Read the model definition and answer for the solid it produces. Units are mm, in the model's axes. A direction names the side the tool comes from. Round coordinates to 2 decimals unless told otherwise and drop trailing zeros. Loops run counter-clockwise (first coordinate to the right, second up) from the corner with the lowest first, then second, coordinate; pieces in that order, holes last. Notation, with made-up numbers: (41.25, -27.5) - (66.25, -27.5) arc R28 ccw to (66.25, 7.5) - close; hole circle Ø11 at (-31.5, 20). An arc over 180 degrees is marked (long way). Use CSV: the item, a comma, the result in double quotes. Start each with the question number.
1. Find section A-A (z = -17). Give the vertices of the cut face in (x, y).
2. Find section B-B (x = 21.5). Give the vertices of the cut face in (y, z).
3. Given pin 1 Ø16.5 at (x, z) = (-16.5, 6.5) entering from -Y, flat-ended and moving along its own axis, determine where the tip first touches the part or whether it passes through.
4. A tool of negligible diameter and unlimited length cuts with its end or side. For faces 1 (the cylindrical face through (7.246, -2.522, -7.744)), 2 (the flat face through (1, 0, -9)), from which of +Z, -Z, +X, -X, +Y, -Y can it reach the whole face along a straight path? Write none if from no direction.
5. Find section D-D (x = -29). Give the vertices of the cut face in (y, z).
6. Find section C-C (z = -34.5). Give the vertices of the cut face in (x, y).
7. Consider line 1 along Z through (x, y) = (8, -1.7); line 2 along X through (y, z) = (-2.4, -21.5); line 3 along Z through (x, y) = (-17.5, -2.7). Determine where each line is inside the solid, lowest interval first.
from build123d import *

# Parameters (mm, degrees)
F0_W     = 76.2
F0_H     = 101.6
F1_DEPTH = 2.54
F2_W     = 33.02
F2_H     = 88.9
F3_DEPTH = 1.27
F4_W     = 17.78
F4_H     = 17.78
F5_DEPTH = 2.54
F6_R     = 2.54
F7_DEPTH = 2.54


with BuildPart() as f1:
    # F0 (on Front) → F1 (new body)
    with BuildSketch(Plane.XZ):
        with Locations((1.335782, -9.618688)):
            Rectangle(F0_W, F0_H)
    extrude(amount=F1_DEPTH)

    # F2 (on face) → F3 (cut)
    with BuildSketch(Plane.XZ.offset(2.54)):
        with Locations((-17.679934, -7.495851)):
            Rectangle(F2_W, F2_H)
        with Locations((20.525211, -7.666058)):
            Rectangle(F2_W, F2_H)
    extrude(amount=-F3_DEPTH, mode=Mode.SUBTRACT)

    # F4 (on face) → F5 (join)
    with BuildSketch(Plane.XZ.offset(1.27)):
        with Locations((-17.624406, 20.281628)):
            Rectangle(F4_W, F4_H)
        with Locations((-17.073924, -4.828554)):
            Rectangle(F4_W, F4_H)
        with Locations((-16.956719, -29.41318)):
            Rectangle(F4_W, F4_H)
        with Locations((20.393534, 20.128676)):
            Rectangle(F4_W, F4_H)
        with Locations((20.905885, -5.264044)):
            Rectangle(F4_W, F4_H)
        with Locations((21.396337, -29.502603)):
            Rectangle(F4_W, F4_H)
    extrude(amount=F5_DEPTH)

    # F6 (on face) → F7 (join)
    with BuildSketch(Plane.XZ.offset(1.27)):
        with Locations((-4.850546, -5.14735)):
            Circle(F6_R)
        with Locations((7.796882, -5.264044)):
            Circle(F6_R)
    extrude(amount=F7_DEPTH)


solid = f1.part
Filled sheet:
1,outline,"(-36.76, -2.54) - (-34.19, -2.54) - (-34.19, -1.27) - (-1.17, -1.27) - (-1.17, -2.54) - (4.02, -2.54) - (4.02, -1.27) - (37.04, -1.27) - (37.04, -2.54) - (39.44, -2.54) - (39.44, 0) - (-36.76, 0) - close"
2,outline,"(-3.81, -38.39) - (-1.27, -38.39) - (-1.27, -52.12) - (-2.54, -52.12) - (-2.54, -60.42) - (0, -60.42) - (0, 41.18) - (-2.54, 41.18) - (-2.54, 36.78) - (-1.27, 36.78) - (-1.27, 29.02) - (-3.81, 29.02) - (-3.81, 11.24) - (-1.27, 11.24) - (-1.27, 3.63) - (-3.81, 3.63) - (-3.81, -14.15) - (-1.27, -14.15) - (-1.27, -20.61) - (-3.81, -20.61) - close"
3,pin 1,"stops at y = -3.81"
4,face 1,"-Y"
4,face 2,"+Z, -Z, +X, -X, +Y"
5,outline,"(-2.54, -60.42) - (0, -60.42) - (0, 41.18) - (-2.54, 41.18) - (-2.54, 36.95) - (-1.27, 36.95) - (-1.27, -51.95) - (-2.54, -51.95) - close"
6,outline,"(-36.76, -2.54) - (-34.19, -2.54) - (-34.19, -1.27) - (-25.85, -1.27) - (-25.85, -3.81) - (-8.07, -3.81) - (-8.07, -1.27) - (-1.17, -1.27) - (-1.17, -2.54) - (4.02, -2.54) - (4.02, -1.27) - (12.51, -1.27) - (12.51, -3.81) - (30.29, -3.81) - (30.29, -1.27) - (37.04, -1.27) - (37.04, -2.54) - (39.44, -2.54) - (39.44, 0) - (-36.76, 0) - close"
7,line 1,"z = -60.42 to -52.12, -7.8 to -2.73, 36.78 to 41.18"
7,line 2,"x = -36.76 to -34.19, -25.85 to -8.07, -1.17 to 4.02, 12.51 to 30.29, 37.04 to 39.44"
7,line 3,"z = -38.3 to -20.52, -13.72 to 4.06, 11.39 to 29.17"
